Geometry: see drawing. Coordinates: mm, zero at the bounding-box minimum. A direction names the side the tool comes from. Round coordinates to 2 decimals unless told otherwise and drop trailing zeros. Write each loop counter-clockwise with the first axis right and the second up, starting at its lowest first coordinate (ties: lowest second). Pieces come first, ordered by that corner, then holes.
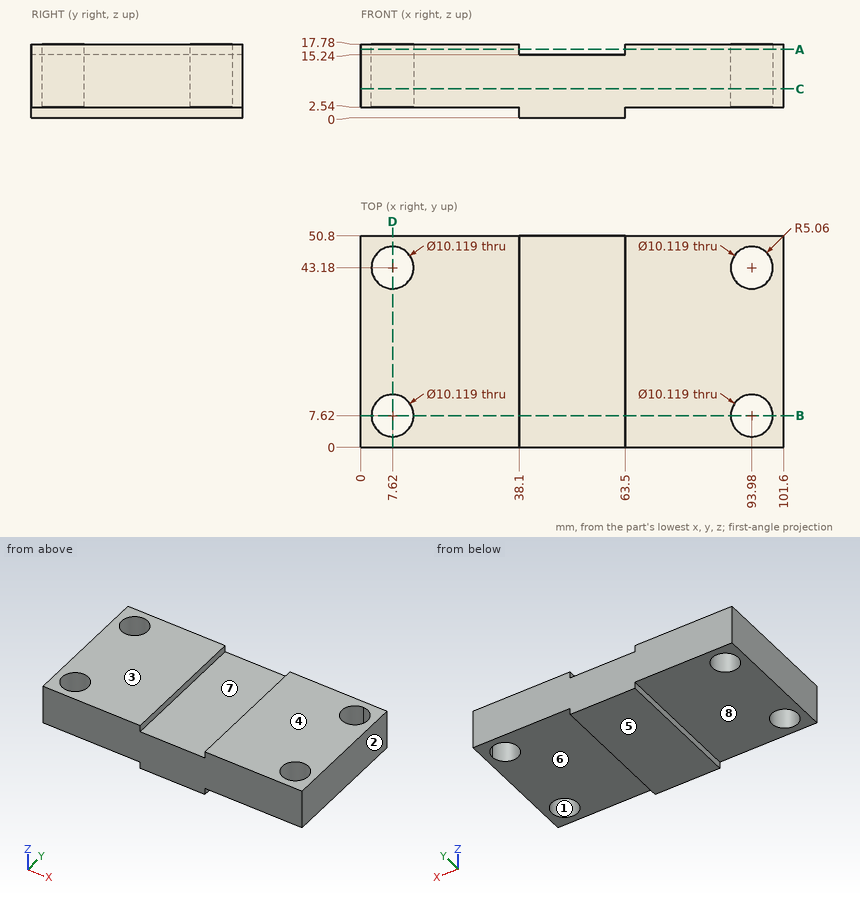
Q1. Mould query, pull axis X, two halves, no side actions, for the marked faces 1, 2 and 3. Classes: pulls with the +X half, pulls with the -X half, needs draft (parallel to the pull), parting line crosses it, or undercut.
Q2. Line query: line 1 (Y direction, x = 93.98, z = 12.5); line 2 (Y direction, x = 89.5, z = 7) (1 decimal); line 3 (X direction, y = 40.5, z = 7.5). Output: solid intervals per line, ascending.
Q3. Section query D-D, the plane x = 7.62. Output: boundary loops of the cut face in (y, z).
Q4. Set-up query: the marked faces 4, 5, 6, 7 and 8. Return all of +Z, -Z, +X, -X, +Y, -Y with unobstructed straight access to the full face (end or side cutting, diameter ignored); none if empty.
Q5. Section query B-B, the plane y = 7.62. Output: boundary loops of the cut face in (x, z), and give its area (3 significant figures).
Q6. Section query A-A, the plane z = 16.5. Output: boundary loops of the cut face in (x, y).
Q7. Pin query (flat end, axial travel): P1, Ø5, axis at y = 15.5, z = 10.5, coming from the -X side; P2, Ø13, axis at x = 93.98, y = 7.62, coming from the -Z side; P3, Ø2, axis at y = 28.5, z = 1, coming from the +X side; P4, Ø2, axis at y = 37, z = 1, coming from the -X side. Return the tip coordinate at first contact, or that it passes through.
Q8. Section query C-C, the plane z = 7. Output: boundary loops of the cut face in (x, y).
Filled in:
1. face 1: undercut
1. face 2: pulls with the +X half
1. face 3: needs draft
2. line 1: y = 0 to 2.56, 12.68 to 38.12, 48.24 to 50.8
2. line 2: y = 0 to 5.3, 10 to 40.8, 45.5 to 50.8
2. line 3: x = 0 to 3.33, 11.91 to 89.69, 98.27 to 101.6
3. outline: (0, 2.54) - (2.56, 2.54) - (2.56, 17.78) - (0, 17.78) - close; (12.68, 2.54) - (38.12, 2.54) - (38.12, 17.78) - (12.68, 17.78) - close; (48.24, 2.54) - (50.8, 2.54) - (50.8, 17.78) - (48.24, 17.78) - close
4. face 4: +Z, +X, -X, +Y, -Y
4. face 5: -Z, +X, -X, +Y, -Y
4. face 6: -Z, +X, +Y, -Y
4. face 7: +Z, +Y, -Y
4. face 8: -Z, -X, +Y, -Y
5. outline: (0, 2.54) - (2.56, 2.54) - (2.56, 17.78) - (0, 17.78) - close; (12.68, 2.54) - (38.1, 2.54) - (38.1, 0) - (63.5, 0) - (63.5, 2.54) - (88.92, 2.54) - (88.92, 17.78) - (63.5, 17.78) - (63.5, 15.24) - (38.1, 15.24) - (38.1, 17.78) - (12.68, 17.78) - close; (99.04, 2.54) - (101.6, 2.54) - (101.6, 17.78) - (99.04, 17.78) - close
5. area: 1,240 mm2
6. outline: (0, 0) - (38.1, 0) - (38.1, 50.8) - (0, 50.8) - close; (63.5, 0) - (101.6, 0) - (101.6, 50.8) - (63.5, 50.8) - close; hole circle Ø10.12 at (7.62, 7.62); hole circle Ø10.12 at (7.62, 43.18); hole circle Ø10.12 at (93.98, 7.62); hole circle Ø10.12 at (93.98, 43.18)
7. P1: stops at x = 0
7. P2: stops at z = 2.54
7. P3: stops at x = 63.5
7. P4: stops at x = 38.1
8. outline: (0, 0) - (101.6, 0) - (101.6, 50.8) - (0, 50.8) - close; hole circle Ø10.12 at (7.62, 7.62); hole circle Ø10.12 at (7.62, 43.18); hole circle Ø10.12 at (93.98, 7.62); hole circle Ø10.12 at (93.98, 43.18)
